Here's how the part is built. I have some questions about the finished solid (model axes, mm). Face numbers are marked on the shaded views. A direction names the side the tool comes from. Coordinates: 2 decimals unless noted, no trailing zeros. Write each loop counter-clockwise with the first axis right and the second up, starting at its lowest first coordinate (ties: lowest second). Pieces come first, ordered by that corner, then holes. Notation, with made-up numbers: (43, 44.5) -> (89, 44.5) arc R33 ccw to (89, 83.5) -> close; hole circle Ø6 at (53.5, -36). An arc over 180 degrees is marked (long way). Put each result on its own line as item: value.
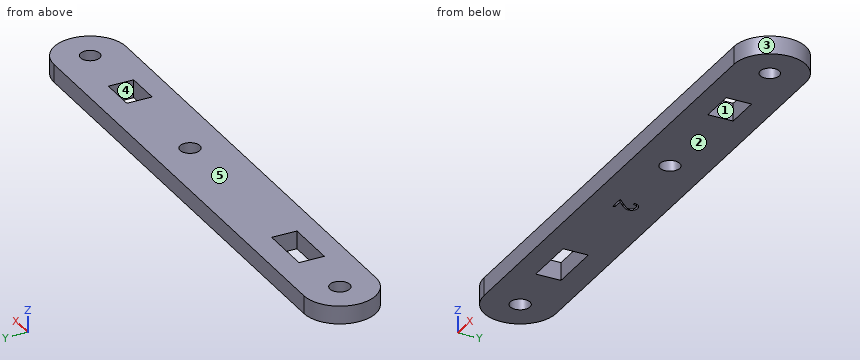
```python
from build123d import *

# Parameters (mm, degrees)
SKETCH_1_R          = 1.65
SKETCH_1_R_2        = 1.3
SKETCH_1_R_3        = 1.6
SKETCH_1_W          = 8.751182885
SKETCH_1_H          = 4.216885397
SKETCH_1_W_2        = 5.900028074
EXTRUDE_1_DEPTH     = 3
SKETCH_2_R          = 1.65
CUT_EXTRUDE_1_DEPTH = 57.708942736
CUT_EXTRUDE_3_DEPTH = 1


with BuildPart() as part:
    # 草图1 → 凸台-拉伸1 (new body)
    with BuildSketch(Plane(origin=(0, 0, 0), x_dir=(-1, 0, 0), z_dir=(0, 0, -1))):
        with BuildLine():
            Line((-30.618171933, 0), (49.343510787, 0))
            ThreePointArc((49.343510787, 0), (55.343510787, 6), (49.343510787, 12))
            Line((49.343510787, 12), (-30.618171933, 12))
            ThreePointArc((-30.618171933, 12), (-36.618171933, 6), (-30.618171933, 0))
        make_face()
        with Locations(Location((49.343510787, 6, 0), (0, 0, 180))):
            Circle(SKETCH_1_R, mode=Mode.SUBTRACT)
        with Locations(Location((1.379286828, 6.00015, 0), (0, 0, 180))):
            Circle(SKETCH_1_R_2, mode=Mode.SUBTRACT)
        with Locations(Location((-30.611606698, 6.0001, 0), (0, 0, 180))):
            Circle(SKETCH_1_R_3, mode=Mode.SUBTRACT)
        with Locations((35.633887137, 5.842992625)):
            Rectangle(SKETCH_1_W, SKETCH_1_H, mode=Mode.SUBTRACT)
        with Locations((-18.07705416, 5.842992625)):
            Rectangle(SKETCH_1_W_2, SKETCH_1_H, mode=Mode.SUBTRACT)
    extrude(amount=-EXTRUDE_1_DEPTH)

    # 草图2 → 切除-拉伸1 (cut, through all)
    with BuildSketch(Plane.XY.offset(3)):
        with Locations((-49.343510787, 6)):
            Circle(SKETCH_2_R)
        with Locations((-1.379286828, 6.00015)):
            Circle(SKETCH_2_R)
    extrude(amount=-CUT_EXTRUDE_1_DEPTH, mode=Mode.SUBTRACT)

    # 草图4 → 切除-拉伸3 (cut)
    with BuildSketch(Plane(origin=(0, 0, 0), x_dir=(-1, 0, 0), z_dir=(0, 0, -1))):
        with BuildLine():
            Line((14.3516244, 6.660828267), (14.037521836, 6.660828267))
            add(Edge.make_bspline(
                [(14.037521836, 6.660828267), (14.039568989, 6.702499155), (14.043589543, 6.78433967), (14.062417832, 6.903663576), (14.089358709, 7.017718375), (14.127450163, 7.125588289), (14.174756441, 7.228227096), (14.231486468, 7.325227112), (14.298680319, 7.4162183), (14.374887053, 7.500357144), (14.457655692, 7.577544715), (14.546961631, 7.644199957), (14.640806659, 7.700517629), (14.738906058, 7.747598871), (14.842366621, 7.782938716), (14.950249479, 7.809160356), (15.063028615, 7.824936702), (15.139868637, 7.826632487), (15.178948118, 7.827494934)],
                knots=[0, 0, 0, 0, 1.10065271, 2.161652631, 3.183658789, 4.190468796, 5.17591951, 6.163126047, 7.15150782, 8.156236427, 9.156009102, 10.134482811, 11.092018607, 12.041330605, 13.001268258, 13.972401359, 14.968799086, 16, 16, 16, 16], degree=3))
            add(Edge.make_bspline(
                [(15.178948118, 7.827494934), (15.217326192, 7.826596478), (15.292737736, 7.824831043), (15.402799751, 7.809670014), (15.507577045, 7.785924422), (15.606864812, 7.752609006), (15.699870876, 7.707824578), (15.787293921, 7.65402704), (15.870174732, 7.591807208), (15.944781515, 7.518553395), (16.013289595, 7.44035101), (16.07239185, 7.356863107), (16.123005013, 7.270633821), (16.165192693, 7.181005619), (16.196248832, 7.087134591), (16.21982704, 6.990387388), (16.233154454, 6.889762577), (16.235199877, 6.821656021), (16.236239784, 6.78703019)],
                knots=[0, 0, 0, 0, 1.111607364, 2.184268762, 3.212621178, 4.221274766, 5.211760367, 6.196651075, 7.1921475, 8.207485113, 9.220403448, 10.201281604, 11.166441695, 12.114753415, 13.065576456, 14.026450734, 14.996634279, 16, 16, 16, 16], degree=3))
            add(Edge.make_bspline(
                [(16.236239784, 6.78703019), (16.234546521, 6.738282356), (16.23118971, 6.641642142), (16.202475333, 6.499627279), (16.157628822, 6.36203386), (16.103631466, 6.251296558), (16.049159021, 6.162063065), (16.000071514, 6.08859436), (15.942606703, 6.009488891), (15.875928205, 5.925011554), (15.801415333, 5.834500649), (15.718393169, 5.738010853), (15.626269687, 5.636539084), (15.561611187, 5.567233482), (15.528106771, 5.531321056)],
                knots=[0, 0, 0, 0, 1.184426356, 2.348067706, 3.509069118, 4.696110526, 5.333549288, 6.050745305, 6.844228056, 7.710549037, 8.667450064, 9.695053472, 10.805634456, 12, 12, 12, 12], degree=3))
            Line((15.528106771, 5.531321056), (14.65240565, 4.596725703))
            Line((14.65240565, 4.596725703), (16.281111579, 4.596725703))
            Line((16.281111579, 4.596725703), (16.281111579, 4.237751344))
            Line((16.281111579, 4.237751344), (13.902906451, 4.237751344))
            Line((13.902906451, 4.237751344), (15.260278246, 5.686268973))
            add(Edge.make_bspline(
                [(15.260278246, 5.686268973), (15.293326133, 5.720767279), (15.35680436, 5.787031466), (15.446586937, 5.883774426), (15.527225925, 5.973523967), (15.599243318, 6.056110515), (15.661076823, 6.132742083), (15.715949055, 6.200936786), (15.759914646, 6.263691237), (15.807630042, 6.336431851), (15.853844023, 6.425244168), (15.893556379, 6.533777857), (15.917771227, 6.64550511), (15.920676063, 6.721007147), (15.92213722, 6.758985319)],
                knots=[0, 0, 0, 0, 1.329631726, 2.553950428, 3.673215718, 4.687767853, 5.603093632, 6.413772471, 7.123043292, 7.734684054, 8.834405432, 9.900288307, 10.943827018, 12, 12, 12, 12], degree=3))
            add(Edge.make_bspline(
                [(15.92213722, 6.758985319), (15.921501478, 6.782866717), (15.920248552, 6.829932367), (15.909190854, 6.898938126), (15.892480348, 6.96550294), (15.86853509, 7.029831559), (15.83692835, 7.091277211), (15.79845497, 7.149914692), (15.754064907, 7.206603657), (15.702713637, 7.259756955), (15.646302118, 7.30843816), (15.586707868, 7.351562246), (15.523657764, 7.387601357), (15.457417642, 7.417144854), (15.388172172, 7.440320235), (15.315787427, 7.456378814), (15.240463411, 7.466461298), (15.189029915, 7.46782547), (15.162822316, 7.468520575)],
                knots=[0, 0, 0, 0, 0.991446411, 1.95395049, 2.89581595, 3.838931463, 4.798493298, 5.75982156, 6.748411868, 7.785213223, 8.824556874, 9.840280684, 10.836137867, 11.835679398, 12.848801643, 13.863922112, 14.911575587, 16, 16, 16, 16], degree=3))
            add(Edge.make_bspline(
                [(15.162822316, 7.468520575), (15.135451484, 7.467805543), (15.081699687, 7.466401338), (15.002780654, 7.456578674), (14.927494877, 7.439632833), (14.855652974, 7.416456159), (14.787133388, 7.38699761), (14.722269344, 7.350305865), (14.661206455, 7.306522372), (14.603829931, 7.256881816), (14.550965952, 7.201614215), (14.504519077, 7.140004251), (14.463935062, 7.073176836), (14.428525829, 7.001312286), (14.399770139, 6.923758506), (14.377796988, 6.840790801), (14.360410142, 6.752769419), (14.354601621, 6.691984334), (14.3516244, 6.660828267)],
                knots=[0, 0, 0, 0, 1.031018746, 2.02475058, 2.990194455, 3.934040569, 4.864654155, 5.795059489, 6.735614925, 7.690564532, 8.649604399, 9.611025574, 10.590972636, 11.591080095, 12.624614302, 13.701020113, 14.821632451, 16, 16, 16, 16], degree=3))
        make_face()
    extrude(amount=-CUT_EXTRUDE_3_DEPTH, mode=Mode.SUBTRACT)


solid = part.part
```
Item 1: Imagine slicing it at B-B on z = 1.8. Write out the boundary of the cut face in (x, y).
Output:
outline: (-49.34, 0) -> (30.62, 0) arc R6 ccw to (30.62, 12) -> (-49.34, 12) arc R6 ccw to start; hole circle Ø3.3 at (-49.34, 6); hole (-40.01, 3.73) -> (-31.26, 3.73) -> (-31.26, 7.95) -> (-40.01, 7.95) -> close; hole circle Ø3.3 at (-1.38, 6); hole (15.13, 3.73) -> (21.03, 3.73) -> (21.03, 7.95) -> (15.13, 7.95) -> close; hole circle Ø3.2 at (30.61, 6)
Item 2: Imagine slicing it at C-C on y = 10. Write out the boundary of the cut face in (x, z).
Output:
outline: (-53.82, 0) -> (35.09, 0) -> (35.09, 3) -> (-53.82, 3) -> close
Item 3: Imagine slicing it at D-D on y = 1.25. Write out the boundary of the cut face in (x, z), then the cut area to 3 significant figures.
Output:
outline: (-53.01, 0) -> (34.28, 0) -> (34.28, 3) -> (-53.01, 3) -> close
area: 262 mm²
Item 4: Imagine slicing it at A-A on x = -37.5. Write out the boundary of the cut face in (y, z).
Output:
outline: (0, 0) -> (3.73, 0) -> (3.73, 3) -> (0, 3) -> close; (7.95, 0) -> (12, 0) -> (12, 3) -> (7.95, 3) -> close
Item 5: If we mould it in two halves opening along X, with no side actions, what happens to the marked faces 1, 2 and 3? For each: released by +X, released by -X, zero draft, split by the parting line, or undercut.
Output:
face 1: undercut
face 2: zero draft
face 3: released by +X
Item 6: Please list where these lines run through material, in increasing order: line 1 along X through (y, z) = (4, 1.9); line 2 along X through (y, z) = (7.75, 2.7); line 3 along X through (y, z) = (5.25, 2.4). Write a range as from..to.
Output:
line 1: x = -55..-40.01, -31.26..15.13, 21.03..36.28
line 2: x = -55.08..-40.01, -31.26..15.13, 21.03..36.36
line 3: x = -55.3..-50.81, -47.87..-40.01, -31.26..-2.85, 0.09..15.13, 21.03..29.2, 32.02..36.57
Item 7: Which directions (+Z, -Z, +X, -X, +Y, -Y) give clear straight access to the entire face, cutting with the end or side of a thin tool? Please do the marked faces 4 and 5.
Output:
face 4: +Z, -Z
face 5: +Z, +X, -X, +Y, -Y
